```python
from build123d import *

# Parameters (mm, degrees)
F1_DEPTH = 76.2
F3_DEPTH = 78.93746
F4_W     = 10.663852
F4_H     = 8.762545
F5_DEPTH = 80.45524
F6_R     = 21.143911
F7_DEPTH = 84.04915


with BuildPart() as f1:
    # F0 (on Front) → F1 (new body)
    with BuildSketch(Plane.XZ):
        Polygon((76.294363, 0), (0, 75.881518), (-75.964086, 0), (-75.964086, -76.376937), (76.294363, -76.376937), align=None)
    extrude(amount=F1_DEPTH)

    # F2 (on Front) → F3 (join)
    with BuildSketch(Plane.XZ):
        Polygon((18.000185, -76.211795), (17.50477, -44.009626), (-14.367121, -44.009626), (-14.367121, -76.211795), align=None)
    extrude(amount=F3_DEPTH)

    # F4 (on Front) → F5 (cut)
    with BuildSketch(Plane.XZ):
        with Locations((-46.53484, -0.088469)):
            Rectangle(F4_W, F4_H)
        with Locations((-35.870988, -0.088469)):
            Rectangle(F4_W, F4_H)
        with Locations((-46.53484, -8.851014)):
            Rectangle(F4_W, F4_H)
        with Locations((-35.870988, -8.851014)):
            Rectangle(F4_W, F4_H)
        with Locations((46.53484, -0.088469)):
            Rectangle(F4_W, F4_H)
        with Locations((46.53484, -8.851014)):
            Rectangle(F4_W, F4_H)
        with Locations((35.870988, -0.088469)):
            Rectangle(F4_W, F4_H)
        with Locations((35.870988, -8.851014)):
            Rectangle(F4_W, F4_H)
    extrude(amount=F5_DEPTH, mode=Mode.SUBTRACT)

    # F6 (on Front) → F7 (cut)
    with BuildSketch(Plane.XZ):
        with Locations((0, 45.625564)):
            Circle(F6_R)
    extrude(amount=F7_DEPTH, mode=Mode.SUBTRACT)


solid = f1.part
```
Here's how the part is built. I have some questions about the finished solid (model axes, mm). A direction names the side the tool comes from. Coordinates: 2 decimals unless noted, no trailing zeros. Loops run counter-clockwise (first coordinate to the right, second up) from the corner with the lowest first, then second, coordinate; pieces in that order, holes last. Notation, with made-up numbers: (69, -5.5) - (100, -5.5) arc R16 ccw to (100, 2.5) - close; hole circle Ø11 at (18, 62.5). An arc over 180 degrees is marked (long way). Return JSON: item names as keys, results as strings. Group by question number.
Item 1: We'd pull the mould along X, two halves only. Please class faces 1 (the face through (-1, 0, -16)), 2 (the face through (-75.964, -38, -38)), 3 (the face through (51.867, -38, -5)): +X half, -X half, draft (parallel to the pull), parting line (faces both ways), or undercut.
Item 2: If we section it at C-C on y = -21: Write out the boundary of the cut face in (x, z), and give its area (3 significant figures).
Item 3: If we section it at A-A on x = -42.5: Write out the boundary of the cut face in (y, z), and give its area (3 significant figures).
Item 4: On a 3-axis mill with a long thin cutter (end or side, diameter ignored), from which of +Z, -Z, +X, -X, +Y, -Y can I reach the whole of each face in a straight line? I mean faces 4 (the face through (38.68, -37.57, 37.41)), 5 (the face through (-51.867, -38, -4)). Say none if no direction works.
Item 5: Will these pins go through, and if not, where does the flat tip stop? P1, Ø0.8, axis at x = -4.5, y = -77.5, coming from the +Z side; P2, Ø6, axis at x = -23.5, z = 55.5, coming from the -Y side; P3, Ø12, axis at y = -70, z = 14, coming from the +X side.
Item 6: If we section it at D-D on x = 25: Write out the boundary of the cut face in (y, z).
Item 7: I need wall thicknesses on line 1 (X direction, y = -62, z = -4); line 2 (Z direction, x = 0, y = -26); line 3 (X direction, y = -24.5, z = 0.5). Which ranges of each line are inside material? Lowest first, please. Write a range as from..to.
Item 8: If we section it at B-B on z = 30.5: Write out the boundary of the cut face in (x, y).
Calculated:
{
 "1": {"face 1": "draft", "face 2": "-X half", "face 3": "undercut"},
 "2": {"outline": "(-75.96, -76.38) - (76.29, -76.38) - (76.29, 0) - (0, 75.88) - (-75.96, 0) - close; hole (-51.87, -13.23) - (-30.54, -13.23) - (-30.54, 4.29) - (-51.87, 4.29) - close; hole circle Ø42.29 at (0, 45.63); hole (30.54, -13.23) - (51.87, -13.23) - (51.87, 4.29) - (30.54, 4.29) - close", "area": "15,300 mm^2"},
 "3": {"outline": "(-76.2, -76.38) - (0, -76.38) - (0, -13.23) - (-76.2, -13.23) - close; (-76.2, 4.29) - (0, 4.29) - (0, 33.43) - (-76.2, 33.43) - close", "area": "7,030 mm^2"},
 "4": {"face 4": "+Z, +X, +Y, -Y", "face 5": "+Y, -Y"},
 "5": {"P1": "stops at z = -44.01", "P2": "stops at y = -76.2", "P3": "stops at x = 68.25"},
 "6": {"outline": "(-76.2, -76.38) - (0, -76.38) - (0, 51.02) - (-76.2, 51.02) - close"},
 "7": {"line 1": "x = -75.96..-51.87, -30.54..30.54, 51.87..76.29", "line 2": "z = -76.38..24.48, 66.77..75.88", "line 3": "x = -75.46..-51.87, -30.54..30.54, 51.87..75.79"},
 "8": {"outline": "(-45.43, -76.2) - (-14.77, -76.2) - (-14.77, 0) - (-45.43, 0) - close; (14.77, -76.2) - (45.63, -76.2) - (45.63, 0) - (14.77, 0) - close"}
}
